Part model, mm, in its own coordinate system. Face numbers are marked on the shaded views. A direction names the side the tool comes from. Round coordinates to 2 decimals unless told otherwise and drop trailing zeros. Write each loop counter-clockwise with the first axis right and the second up, starting at its lowest first coordinate (ties: lowest second). Pieces come first, ordered by that corner, then holes. Notation, with made-up numbers: M 9,43 L 15,43 A17 ccw 15,49 Z; hole C -6,48.5 d9. An arc over 180 degrees is marked long. Use a Markdown table: item, result. Add a question column.
1) Slice it at B-B on z = 1.5. Write the cut outline in (x, y) (3 decimals).
2) Slice it at D-D on y = -37.5. Write the cut outline in (x, z), plus the area to 3 significant figures.
3) Which spindle directions (+Z, -Z, +X, -X, +Y, -Y) get a long thin tool onto all of the face, cutting with end or side? Do the marked faces 1 and 2. Say none if no direction does.
4) Drop flat-ended pins along their axis: P1, Ø2, axis at y = -21, z = -24, coming from the +X side; P2, Ø9, axis at y = -15.88, z = -22, coming from the +X side; P3, Ø3.5, axis at y = -31.75, z = -22, coming from the +X side; P4, Ø2, axis at y = -38.5, z = 18, coming from the -X side. Give the stop position or say it passes through.
5) Slice it at C-C on x = 31. Write the cut outline in (y, z), plus the area to 3 significant figures.
6) Wall check: probe 1 along X at (y, z) = (-15, 2.5); probe 2 along Y at (x, z) = (21.5, 3). Give the ranges that are in metal, low to high.
7) Slice it at A-A on y = -44.45. Write the cut outline in (x, z), plus the area to 3 significant figures.
```python
from build123d import *

# Parameters (mm, degrees)
EXTRUDE1_DEPTH                  = 38.1
F_7_32_0_21875_DIAMETER_HOLE2_D = 5.55625
F_7_32_0_21875_DIAMETER_HOLE3_D = 5.55625
SKETCH6_R                       = 6.35
CUT_EXTRUDE1_DEPTH              = 9.525


with BuildPart() as part:
    # Sketch1 → Extrude1 (new body, symmetric)
    with BuildSketch(Plane.XY):
        with BuildLine():
            Line((0, 0), (50.8, 0))
            Line((50.8, 0), (50.8, -3.175))
            ThreePointArc((50.8, -3.175), (49.87006403, -5.42006403), (47.625, -6.35))
            Line((47.625, -6.35), (12.7, -6.35))
            ThreePointArc((12.7, -6.35), (8.209871939, -8.209871939), (6.35, -12.7))
            Line((6.35, -12.7), (6.35, -47.625))
            ThreePointArc((6.35, -47.625), (5.42006403, -49.87006403), (3.175, -50.8))
            Line((3.175, -50.8), (0, -50.8))
            Line((0, -50.8), (0, 0))
        make_face()
    extrude(amount=EXTRUDE1_DEPTH, both=True)

    # 7/32 (0.21875) Diameter Hole2 (through all)
    with Locations(Plane(origin=(-45.24375, 0, 38.1), x_dir=(-1, 0, 0), z_dir=(0, 1, 0))):
        with Locations((-84.93125, -19.05), (-84.93125, -57.15), (-59.53125, -57.15), (-59.53125, -19.05)):
            Hole(F_7_32_0_21875_DIAMETER_HOLE2_D / 2)

    # 7/32 (0.21875) Diameter Hole3 (through all)
    with Locations(Plane(origin=(6.35, 0, 0), x_dir=(0, 0, -1), z_dir=(1, 0, 0))):
        with Locations((-21.9964, -15.875), (21.9964, -15.875), (21.9964, -44.45), (-21.9964, -44.45), (-21.9964, -31.75), (21.9964, -31.75)):
            Hole(F_7_32_0_21875_DIAMETER_HOLE3_D / 2)

    # Sketch6 → Cut-Extrude1 (cut)
    with BuildSketch(Plane(origin=(0, -15.875, 0), x_dir=(-1, 0, 0), z_dir=(0, 1, 0))):
        with Locations((-14.2875, 19.05)):
            Circle(SKETCH6_R)
        with Locations((-14.2875, -19.05)):
            Circle(SKETCH6_R)
    extrude(amount=CUT_EXTRUDE1_DEPTH, mode=Mode.SUBTRACT)


solid = part.part
```
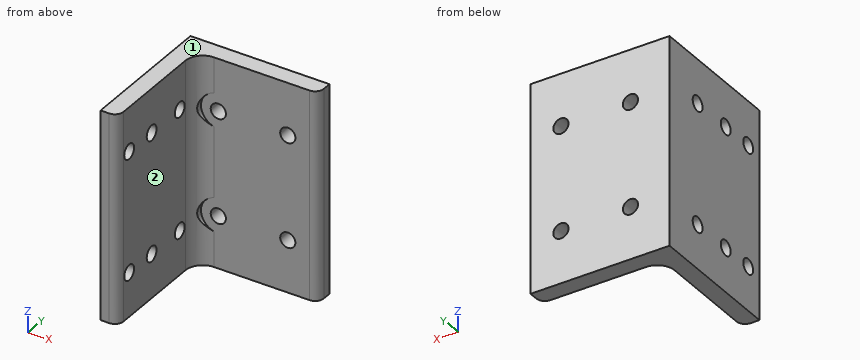
Entries:
| question | item | result |
|---|---|---|
| 1 | outline | M 0,-50.8 L 3.175,-50.8 A3.175 ccw 6.35,-47.625 L 6.35,-12.7 A6.35 cw 12.7,-6.35 L 47.625,-6.35 A3.175 ccw 50.8,-3.175 L 50.8,0 L 0,0 Z |
| 2 | outline | M 0,-38.1 L 6.35,-38.1 L 6.35,38.1 L 0,38.1 Z |
| 2 | area | 484 mm^2 |
| 3 | face 1 | +Z, +X, -X, +Y, -Y |
| 3 | face 2 | +Z, -Z, +X, -Y |
| 4 | P1 | stops at x = 6.35 |
| 4 | P2 | stops at x = 6.49 |
| 4 | P3 | passes through |
| 4 | P4 | stops at x = 0 |
| 5 | outline | M -6.35,-38.1 L 0,-38.1 L 0,38.1 L -6.35,38.1 Z |
| 5 | area | 484 mm^2 |
| 6 | probe 1 | x = 0 to 6.35 |
| 6 | probe 2 | y = -6.35 to 0 |
| 7 | outline | M 0,-38.1 L 6.35,-38.1 L 6.35,-24.77 L 0,-24.77 Z; M 0,-19.22 L 6.35,-19.22 L 6.35,19.22 L 0,19.22 Z; M 0,24.77 L 6.35,24.77 L 6.35,38.1 L 0,38.1 Z |
| 7 | area | 413 mm^2 |
